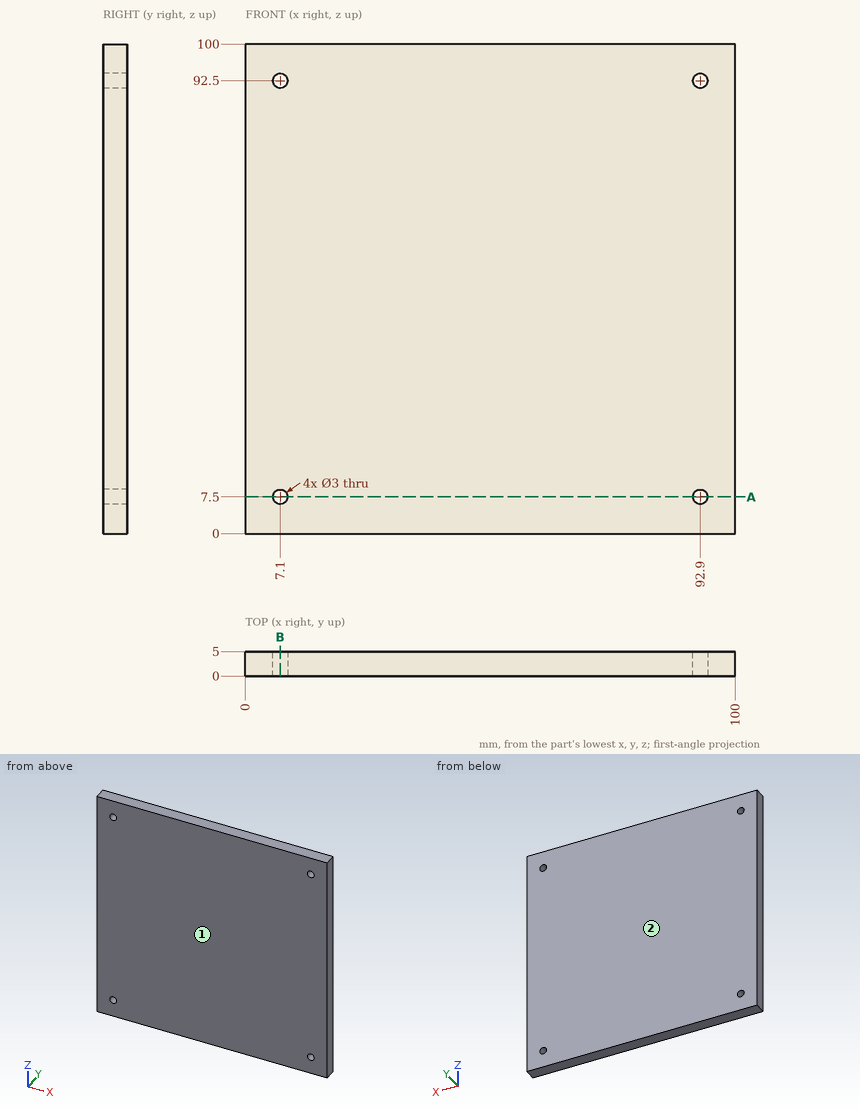
Part print with two shaded views. Sizes in mm from the minimum x, y, z corner. Round coordinates to 2 decimals unless told otherwise and drop trailing zeros. Order: outer loops, then holes, each group sorted by start corner. A loop starts at its lowest first (then second) coordinate and runs counter-clockwise, first axis right, second up. Notation, with made-up numbers: M 50.5,61.5 L 104.5,61.5 A19 cw 104.5,69.5 Z; hole C -33,36 d9. An arc over 180 degrees is marked long. Use CSV: the item, a comma, the result in double quotes. Start each with the question number.
(1) Mould opens along Y. For the marked faces 1 and 2 say: +Y half, -Y half, draft (parallel to the pull), parting line (faces both ways), or undercut.
(2) Cut at A-A on z = 7.5. List the corners of the cut face in (x, y).
(3) Cut at B-B on x = 7.1. List the corners of the cut face in (y, z), then the cut area to 3 significant figures.
(4) Drill centre lines: probe 1 along X at (y, z) = (2.1, 92.5); probe 2 along Z at (x, y) = (92.9, 1.55). Where is each one in solid material? Low to high.
(5) Flat gauge pin, fed straight in: P1, Ø1.8, axis at x = 92.9, z = 7.5, coming from the -Y side. Where does the tip first touch, or does it go through?
Findings:
1,face 1,"-Y half"
1,face 2,"+Y half"
2,outline,"M 0,0 L 5.6,0 L 5.6,5 L 0,5 Z; M 8.6,0 L 91.4,0 L 91.4,5 L 8.6,5 Z; M 94.4,0 L 100,0 L 100,5 L 94.4,5 Z"
3,outline,"M 0,0 L 5,0 L 5,6 L 0,6 Z; M 0,9 L 5,9 L 5,91 L 0,91 Z; M 0,94 L 5,94 L 5,100 L 0,100 Z"
3,area,"470 mm^2"
4,probe 1,"x = 0 to 5.6, 8.6 to 91.4, 94.4 to 100"
4,probe 2,"z = 0 to 6, 9 to 91, 94 to 100"
5,P1,"passes through"
